Build history of the part. All positions in model axes, mm. Face numbers are marked on the shaded views. A direction names the side the tool comes from. Coordinates: 2 decimals unless noted, no trailing zeros. Loops run counter-clockwise (first coordinate to the right, second up) from the corner with the lowest first, then second, coordinate; pieces in that order, holes last.
(1) Flat gauge pins, fed straight in: P1, Ø2, axis at x = 111, z = 24.5, coming from the +Y side; P2, Ø5, axis at y = 9, z = 210, coming from the +X side; P3, Ø5, axis at y = 151, z = 73.5, coming from the -X side. Where does each tip first touch, or does it go through?
(2) Slice it at D-D (y = 176). Give the number of separate pieces and of enclosed holes in the cut face, and give its area (3 significant figures).
(3) Wall check: L1, parallel to Y at x = 195.5, z = 209; L2, parallel to Z at x = 118, y = 97.5; L3, parallel to X at y = 37, z = -20. Give the ranges that are in metal, low to high.
(4) Slice it at A-A (y = 56). Give the cut face in (x, z).
(5) Tool access for the marked faces 1, 2 and 3: list every direction of +Z, -Z, +X, -X, +Y, -Y with a clear straight run to the whole face (end or side of a thin tool).
(6) Slice it at B-B (z = 156). Give the cut face in (x, y).
(7) Slice it at C-C (x = 147). Give the cut face in (y, z), and give its area (3 significant figures).
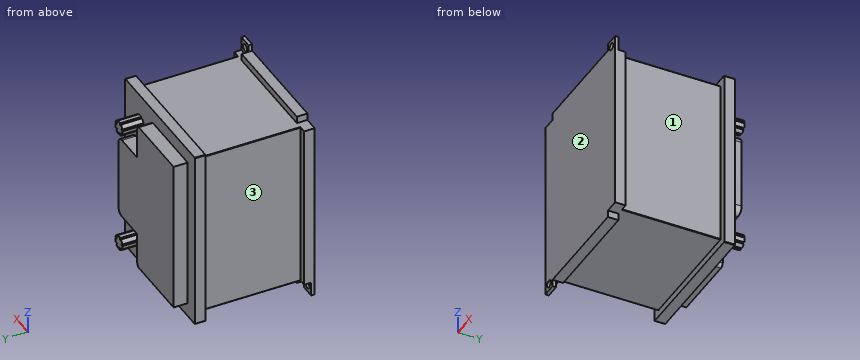
from build123d import *

# Parameters (mm, degrees)
SKETCH1_W           = 172
SKETCH1_H           = 239
BOSS_EXTRUDE1_DEPTH = 190
SKETCH2_W           = 172
SKETCH2_H           = 239
SKETCH2_W_2         = 152
SKETCH2_H_2         = 219
CUT_EXTRUDE1_DEPTH  = 20
SKETCH3_W           = 52
SKETCH3_H           = 50
CUT_EXTRUDE2_DEPTH  = 20
FILLET1_R           = 10
FILLET2_R           = 10
FILLET3_R           = 5
FILLET4_R           = 5
FILLET6_R           = 1
FILLET7_R           = 1
FILLET8_R           = 1
FILLET9_R           = 1
SKETCH4_R           = 10
BOSS_EXTRUDE4_DEPTH = 30
CUT_EXTRUDE8_START  = -30
CUT_EXTRUDE8_DEPTH  = 30
CUT_EXTRUDE9_START  = -30
CUT_EXTRUDE9_DEPTH  = 30
BOSS_EXTRUDE5_DEPTH = 15
SKETCH11_W          = 20
SKETCH11_H          = 10
CUT_EXTRUDE11_DEPTH = 15
SKETCH12_W          = 20
SKETCH12_H          = 5
BOSS_EXTRUDE6_DEPTH = 20
SKETCH13_R          = 5
CUT_EXTRUDE12_DEPTH = 20
SKETCH14_W          = 20
SKETCH14_H          = 5
BOSS_EXTRUDE7_DEPTH = 20
SKETCH15_R          = 5
CUT_EXTRUDE13_DEPTH = 20


with BuildPart() as part:
    # Sketch1 → Boss-Extrude1 (new body)
    with BuildSketch(Plane(origin=(0, 0, 0), x_dir=(1, 0, 0), z_dir=(0, 1, 0))):
        with Locations((116.427433091, -83.803086818)):
            Rectangle(SKETCH1_W, SKETCH1_H)
    extrude(amount=BOSS_EXTRUDE1_DEPTH)

    # Sketch2 → Cut-Extrude1 (cut)
    with BuildSketch(Plane(origin=(0, 190, 0), x_dir=(1, 0, 0), z_dir=(0, 1, 0))):
        with Locations((116.427433091, -83.803086818)):
            Rectangle(SKETCH2_W, SKETCH2_H)
        with Locations((116.427433091, -83.803086818)):
            Rectangle(SKETCH2_W_2, SKETCH2_H_2, mode=Mode.SUBTRACT)
    extrude(amount=-CUT_EXTRUDE1_DEPTH, mode=Mode.SUBTRACT)

    # Sketch3 → Cut-Extrude2 (cut)
    with BuildSketch(Plane(origin=(0, 190, 0), x_dir=(1, 0, 0), z_dir=(0, 1, 0))):
        with Locations((166.427433091, 0.696913182)):
            Rectangle(SKETCH3_W, SKETCH3_H)
        with Locations((166.427433091, -168.303086818)):
            Rectangle(SKETCH3_W, SKETCH3_H)
    extrude(amount=-CUT_EXTRUDE2_DEPTH, mode=Mode.SUBTRACT)

    # Fillet1
    fillet1_edges = [part.edges().sort_by_distance(p)[0] for p in [
        (192.427433091, 180, 24.303086818),
    ]]
    fillet(fillet1_edges, radius=FILLET1_R)

    # Fillet2
    fillet2_edges = [part.edges().sort_by_distance(p)[0] for p in [
        (192.427433091, 180, 143.303086818),
    ]]
    fillet(fillet2_edges, radius=FILLET2_R)

    # Fillet3
    fillet3_edges = [part.edges().sort_by_distance(p)[0] for p in [
        (140.427433091, 180, 193.303086818),
    ]]
    fillet(fillet3_edges, radius=FILLET3_R)

    # Fillet4
    fillet4_edges = [part.edges().sort_by_distance(p)[0] for p in [
        (140.427433091, 180, -25.696913182),
    ]]
    fillet(fillet4_edges, radius=FILLET4_R)

    # Fillet6
    fillet6_edges = [part.edges().sort_by_distance(p)[0] for p in [
        (30.427433091, 85, 203.303086818),
    ]]
    fillet(fillet6_edges, radius=FILLET6_R)

    # Fillet7
    fillet7_edges = [part.edges().sort_by_distance(p)[0] for p in [
        (202.427433091, 85, 203.303086818),
    ]]
    fillet(fillet7_edges, radius=FILLET7_R)

    # Fillet8
    fillet8_edges = [part.edges().sort_by_distance(p)[0] for p in [
        (202.427433091, 85, -35.696913182),
    ]]
    fillet(fillet8_edges, radius=FILLET8_R)

    # Fillet9
    fillet9_edges = [part.edges().sort_by_distance(p)[0] for p in [
        (30.427433091, 85, -35.696913182),
    ]]
    fillet(fillet9_edges, radius=FILLET9_R)

    # Sketch4 → Boss-Extrude4 (add)
    with BuildSketch(Plane(origin=(0, 170, 0), x_dir=(1, 0, 0), z_dir=(0, 1, 0))):
        with Locations(Location((171.427433091, -172.803086818, 0), (0, 0, 270))):
            Circle(SKETCH4_R)
        with Locations(Location((171.427433091, 5.696913182, 0), (0, 0, 270))):
            Circle(SKETCH4_R)
    extrude(amount=BOSS_EXTRUDE4_DEPTH)

    # Sketch7 → Cut-Extrude8 (cut)
    with BuildSketch(Plane(origin=(0, 200, 0), x_dir=(1, 0, 0), z_dir=(0, 1, 0)).offset(CUT_EXTRUDE8_START)):
        with BuildLine():
            Line((166.237215884, -167.741646234), (164.26810659, -165.821393323))
            ThreePointArc((164.26810659, -165.821393323), (163.503030714, -166.703591185), (162.846013112, -167.668962633))
            Line((162.846013112, -167.668962633), (165.181081901, -169.06599636))
            Line((165.181081901, -169.06599636), (166.237215884, -167.741646234))
        make_face()
        with BuildLine():
            Line((164.234191998, -173.705205444), (161.505158254, -174.047458976))
            ThreePointArc((161.505158254, -174.047458976), (161.71787131, -175.195660752), (162.062985325, -176.31123705))
            Line((162.062985325, -176.31123705), (164.611121852, -175.35664304))
            Line((164.611121852, -175.35664304), (164.234191998, -173.705205444))
        make_face()
        with BuildLine():
            Line((167.647825369, -178.989450929), (166.213885247, -181.336487013))
            ThreePointArc((166.213885247, -181.336487013), (167.244209965, -181.886073347), (168.331577706, -182.31180279))
            Line((168.331577706, -182.31180279), (169.173983194, -179.724409801))
            Line((169.173983194, -179.724409801), (167.647825369, -178.989450929))
        make_face()
        with BuildLine():
            ThreePointArc((174.848520104, -182.199690654), (175.920600956, -181.736811827), (176.931412335, -181.15211146))
            Line((176.931412335, -181.15211146), (175.433738269, -178.880279187))
            Line((175.433738269, -178.880279187), (173.907580445, -179.61523806))
            Line((173.907580445, -179.61523806), (174.848520104, -182.199690654))
        make_face()
        with BuildLine():
            ThreePointArc((180.907006662, -175.987059951), (181.2135449, -174.86027316), (181.386638332, -173.705434286))
            Line((181.386638332, -173.705434286), (178.676663832, -173.459898767))
            Line((178.676663832, -173.459898767), (178.299733977, -175.111336363))
            Line((178.299733977, -175.111336363), (180.907006662, -175.987059951))
        make_face()
        with BuildLine():
            ThreePointArc((179.827180973, -167.376832537), (179.137347052, -166.434631219), (178.342379652, -165.579271064))
            Line((178.342379652, -165.579271064), (176.460770789, -167.544925553))
            Line((176.460770789, -167.544925553), (177.516904772, -168.869275679))
            Line((177.516904772, -168.869275679), (179.827180973, -167.376832537))
        make_face()
        with BuildLine():
            ThreePointArc((172.422173805, -162.852685273), (171.255426737, -162.804566237), (170.091025172, -162.892788443))
            Line((170.091025172, -162.892788443), (170.454671798, -165.589455018))
            Line((170.454671798, -165.589455018), (172.148579189, -165.589455018))
            Line((172.148579189, -165.589455018), (172.422173805, -162.852685273))
        make_face()
    extrude(amount=CUT_EXTRUDE8_DEPTH, mode=Mode.SUBTRACT)

    # Sketch8 → Cut-Extrude9 (cut)
    with BuildSketch(Plane(origin=(0, 200, 0), x_dir=(1, 0, 0), z_dir=(0, 1, 0)).offset(CUT_EXTRUDE9_START)):
        with BuildLine():
            Line((166.375783325, 11.009561317), (164.536616638, 12.943750328))
            ThreePointArc((164.536616638, 12.943750328), (163.767883793, 12.125855906), (163.095653722, 11.226963141))
            Line((163.095653722, 11.226963141), (165.353867519, 9.728119429))
            Line((165.353867519, 9.728119429), (166.375783325, 11.009561317))
        make_face()
        with BuildLine():
            ThreePointArc((172.796884735, 15.60269948), (171.678132038, 15.69377019), (170.55622078, 15.658890351))
            Line((170.55622078, 15.658890351), (170.792350852, 12.95883394))
            Line((170.792350852, 12.95883394), (172.431376546, 12.95883394))
            Line((172.431376546, 12.95883394), (172.796884735, 15.60269948))
        make_face()
        with BuildLine():
            ThreePointArc((180.025927812, 10.802389509), (179.399598862, 11.733847248), (178.672828478, 12.589245565))
            Line((178.672828478, 12.589245565), (176.709064064, 10.721174005))
            Line((176.709064064, 10.721174005), (177.730979869, 9.439732117))
            Line((177.730979869, 9.439732117), (180.025927812, 10.802389509))
        make_face()
        with BuildLine():
            ThreePointArc((180.780128986, 2.15755173), (181.117862258, 3.227989823), (181.33350567, 4.329533917))
            Line((181.33350567, 4.329533917), (178.648601427, 4.700143193))
            Line((178.648601427, 4.700143193), (178.283883899, 3.102211295))
            Line((178.283883899, 3.102211295), (180.780128986, 2.15755173))
        make_face()
        with BuildLine():
            Line((164.124185412, 5.059756289), (161.465273877, 4.827784996))
            ThreePointArc((161.465273877, 4.827784996), (161.625432396, 3.716816625), (161.909086465, 2.63079552))
            Line((161.909086465, 2.63079552), (164.48890294, 3.461824392))
            Line((164.48890294, 3.461824392), (164.124185412, 5.059756289))
        make_face()
        with BuildLine():
            Line((167.37208196, -0.410256602), (165.895640195, -2.633709085))
            ThreePointArc((165.895640195, -2.633709085), (166.864087446, -3.201169563), (167.890028356, -3.656522965))
            Line((167.890028356, -3.656522965), (168.848793084, -1.121403199))
            Line((168.848793084, -1.121403199), (167.37208196, -0.410256602))
        make_face()
        with BuildLine():
            ThreePointArc((174.491559391, -3.822074685), (175.539034842, -3.418717956), (176.534708162, -2.900513255))
            Line((176.534708162, -2.900513255), (175.150451748, -0.570299486))
            Line((175.150451748, -0.570299486), (173.673740624, -1.281446083))
            Line((173.673740624, -1.281446083), (174.491559391, -3.822074685))
        make_face()
    extrude(amount=CUT_EXTRUDE9_DEPTH, mode=Mode.SUBTRACT)

    # Sketch9 → Boss-Extrude5 (add)
    with BuildSketch(Plane(origin=(0, 170, 0), x_dir=(1, 0, 0), z_dir=(0, 1, 0))):
        with BuildLine():
            Line((21.427433091, 45.696913182), (211.427433091, 45.696913182))
            ThreePointArc((211.427433091, 45.696913182), (212.134539872, 45.404019963), (212.427433091, 44.696913182))
            Line((212.427433091, 44.696913182), (212.427433091, -212.303086818))
            ThreePointArc((212.427433091, -212.303086818), (212.134539872, -213.010193599), (211.427433091, -213.303086818))
            Line((211.427433091, -213.303086818), (21.427433091, -213.303086818))
            ThreePointArc((21.427433091, -213.303086818), (20.720326309, -213.010193599), (20.427433091, -212.303086818))
            Line((20.427433091, -212.303086818), (20.427433091, 44.696913182))
            ThreePointArc((20.427433091, 44.696913182), (20.720326309, 45.404019963), (21.427433091, 45.696913182))
        make_face()
        with BuildLine():
            Line((31.427433091, 35.696913182), (201.427433091, 35.696913182))
            ThreePointArc((201.427433091, 35.696913182), (202.134539872, 35.404019963), (202.427433091, 34.696913182))
            Line((202.427433091, 34.696913182), (202.427433091, -202.303086818))
            ThreePointArc((202.427433091, -202.303086818), (202.134539872, -203.010193599), (201.427433091, -203.303086818))
            Line((201.427433091, -203.303086818), (31.427433091, -203.303086818))
            ThreePointArc((31.427433091, -203.303086818), (30.720326309, -203.010193599), (30.427433091, -202.303086818))
            Line((30.427433091, -202.303086818), (30.427433091, 34.696913182))
            ThreePointArc((30.427433091, 34.696913182), (30.720326309, 35.404019963), (31.427433091, 35.696913182))
        make_face(mode=Mode.SUBTRACT)
    boss_extrude5 = extrude(amount=-BOSS_EXTRUDE5_DEPTH)

    # Mirror2: Boss-Extrude5 across plane
    add(boss_extrude5.mirror(Plane.ZX.offset(85)))

    # Sketch11 → Cut-Extrude11 (cut)
    with BuildSketch(Plane(origin=(0, 15, 0), x_dir=(1, 0, 0), z_dir=(0, 1, 0))):
        with Locations((30.427433091, -208.303086818)):
            Rectangle(SKETCH11_W, SKETCH11_H)
        with Locations((202.427433091, -208.303086818)):
            Rectangle(SKETCH11_W, SKETCH11_H)
        with Locations((202.427433091, 40.696913182)):
            Rectangle(SKETCH11_W, SKETCH11_H)
        with Locations((30.427433091, 40.696913182)):
            Rectangle(SKETCH11_W, SKETCH11_H)
    extrude(amount=-CUT_EXTRUDE11_DEPTH, mode=Mode.SUBTRACT)

    # Sketch12 → Boss-Extrude6 (add)
    with BuildSketch(Plane.XY.offset(203.303086818)):
        with Locations((202.427433091, 2.5)):
            Rectangle(SKETCH12_W, SKETCH12_H)
    extrude(amount=BOSS_EXTRUDE6_DEPTH)

    # Sketch13 → Cut-Extrude12 (cut)
    with BuildSketch(Plane(origin=(0, 5, 0), x_dir=(1, 0, 0), z_dir=(0, 1, 0))):
        with Locations(Location((202.427433091, -213.303086818, 0), (0, 0, 270))):
            Circle(SKETCH13_R)
    extrude(amount=-CUT_EXTRUDE12_DEPTH, mode=Mode.SUBTRACT)

    # Sketch14 → Boss-Extrude7 (add)
    with BuildSketch(Plane(origin=(0, 0, -35.696913182), x_dir=(-1, 0, 0), z_dir=(0, 0, -1))):
        with Locations((-30.427433091, 2.5)):
            Rectangle(SKETCH14_W, SKETCH14_H)
    extrude(amount=BOSS_EXTRUDE7_DEPTH)

    # Sketch15 → Cut-Extrude13 (cut)
    with BuildSketch(Plane(origin=(0, 5, 0), x_dir=(1, 0, 0), z_dir=(0, 1, 0))):
        with Locations(Location((30.427433091, 45.696913182, 0), (0, 0, 270))):
            Circle(SKETCH15_R)
    extrude(amount=-CUT_EXTRUDE13_DEPTH, mode=Mode.SUBTRACT)


solid = part.part
Response values:
1. P1: stops at y = 190
1. P2: stops at x = 192.43
1. P3: stops at x = 30.43
2. separate pieces: 3
2. enclosed holes: 0
2. area: 28,600 mm2
3. L1: y = 0 to 5, 155 to 170
3. L2: z = -35.7 to 203.3
3. L3: x = 30.43 to 202.43
4. outline: (30.43, -34.7) arc R1 ccw to (31.43, -35.7) - (201.43, -35.7) arc R1 ccw to (202.43, -34.7) - (202.43, 202.3) arc R1 ccw to (201.43, 203.3) - (31.43, 203.3) arc R1 ccw to (30.43, 202.3) - close
5. face 1: +Z, -Z, +X
5. face 2: +Z, -Z, +X, -X, -Y
5. face 3: +Z, -Z, -X
6. outline: (20.43, 0) - (212.43, 0) - (212.43, 15) - (202.43, 15) - (202.43, 155) - (212.43, 155) - (212.43, 170) - (140.43, 170) - (140.43, 190) - (40.43, 190) - (40.43, 170) - (20.43, 170) - (20.43, 155) - (30.43, 155) - (30.43, 15) - (20.43, 15) - close
7. outline: (0, -45.7) - (15, -45.7) - (15, -35.7) - (155, -35.7) - (155, -45.7) - (170, -45.7) - (170, 24.3) - (190, 24.3) - (190, 143.3) - (170, 143.3) - (170, 213.3) - (155, 213.3) - (155, 203.3) - (15, 203.3) - (15, 213.3) - (0, 213.3) - close
7. area: 43,600 mm2
